Input: part model. Units: mm. Frame: model coordinates. Coordinates: 2 decimals unless noted, no trailing zeros. Order: outer loops, then holes, each group sorted by start corner. A loop starts at its lowest first (then second) coordinate and runs counter-clockwise, first axis right, second up. Notation, with made-up numbers: (-34, 54) - (15, 54) arc R8 ccw to (15, 59) - close; hole circle Ø9 at (64.25, 60.5). An arc over 180 degrees is marked (long way). One line per question, with ' | ' between items. Start each with the question number.
```python
from build123d import *

# Parameters (mm, degrees)
REVOLVE3_ANGLE      = 90
BOSS_EXTRUDE2_DEPTH = 1000
BOSS_EXTRUDE4_DEPTH = 50


with BuildPart() as part:
    # Sketch2 → Revolve3 (revolve)
    with BuildSketch(Plane.XY):
        with BuildLine():
            Line((-0.654182434, 15.02), (-10.654182434, 15.02))
            Line((-10.654182434, 15.02), (-10.654182434, 0))
            Line((-10.654182434, 0), (0, 0))
            Line((0, 0), (25.4, 0))
            Line((25.4, 0), (35.4, 0))
            Line((35.4, 0), (35.4, 4.5))
            Line((35.4, 4.5), (25.4, 4.5))
            add(Edge.make_bspline(
                [(-0.654182434, 15.02), (-0.219836229, 14.810704372), (0.610598489, 14.410982375), (2.74095302, 13.386545583), (4.34709547, 12.619135975), (6.701613478, 11.49599419), (8.606916476, 10.59589253), (10.790885987, 9.570629713), (12.810835282, 8.63757915), (14.944119423, 7.669787097), (16.950761864, 6.79193378), (18.75556814, 6.044207346), (20.238794329, 5.486207444), (21.39416777, 5.103578745), (22.215591012, 4.870934478), (22.897035956, 4.710298297), (23.464492683, 4.605633048), (23.954091395, 4.538072471), (24.354277235, 4.503624983), (24.669284768, 4.488813447), (24.918595629, 4.485402054), (25.124701431, 4.488218611), (25.279381224, 4.493757229), (25.359889237, 4.497669109), (25.4, 4.5)],
                knots=[0.083771138, 0.083771138, 0.083771138, 0.083771138, 0.083771138, 0.152014176, 0.220257214, 0.288500251, 0.356743288, 0.424986327, 0.493229366, 0.561472406, 0.629715448, 0.697958493, 0.757156968, 0.791278497, 0.81934393, 0.841893906, 0.858954658, 0.874282948, 0.887931591, 0.900718778, 0.906405686, 0.912092593, 0.917779499, 0.923466404, 0.923466404, 0.923466404, 0.923466404, 0.923466404], degree=4))
        make_face()
    revolve(axis=Axis((0, 0, 0), (1, 0, 0)), revolution_arc=REVOLVE3_ANGLE)

    # Sketch11 → Boss-Extrude2 (add)
    with BuildSketch(Plane.XY):
        with BuildLine():
            Line((25.133318649, 0), (101.333318649, 0))
            ThreePointArc((101.333318649, 0), (63.233318649, 38.1), (25.133318649, 0))
        make_face()
    extrude(amount=BOSS_EXTRUDE2_DEPTH)

    # Sketch16 → Boss-Extrude4 (add)
    with BuildSketch(Plane(origin=(0, 0, 0), x_dir=(0, 0, -1), z_dir=(1, 0, 0))):
        with BuildLine():
            Line((-967.503760297, 0), (-970.507760297, 0))
            ThreePointArc((-970.507760297, 0), (-969.005760297, 1.502), (-967.503760297, 0))
        make_face()
    extrude(amount=BOSS_EXTRUDE4_DEPTH)


solid = part.part
```
(1) Material intervals for line 1 along X through (y, z) = (3.5, 347); line 2 along Y through (x, z) = (59.5, 267.5); line 3 along Y through (x, z) = (60, 129), sorted ascending. Write a range as from..to.
(2) Section B-B (x = 51). Output: boundary loops of the cut face in (y, z), then the cut area to 3 significant figures.
(3) Section A-A (z = 776). Output: boundary loops of the cut face in (x, y), then the cut area to 3 significant figures.
(4) Section C-C (y = 29). Output: boundary loops of the cut face in (x, z).
(5) Pin query (flat end, axial travel): pin 1 (1.5 mm diameter, centred on y = 20, z = 176.5, fed in from -X); pin 2 (12 mm diameter, centred on x = 59, z = 537, fed in from +Y); pin 3 (1.2 mm diameter, centred on y = 1, z = 969, fed in from -X). Return the tip coordinate at first contact, or that it passes through.
Worked answers:
1) line 1: x = 25.29..101.17 | line 2: y = 0..37.92 | line 3: y = 0..37.96
2) outline: (0, 0) - (36.08, 0) - (36.08, 1000) - (0, 1000) - close | area: 36,100 mm²
3) outline: (25.13, 0) - (101.33, 0) arc R38.1 ccw to start | area: 2,280 mm²
4) outline: (38.52, 0) - (87.94, 0) - (87.94, 1000) - (38.52, 1000) - close
5) pin 1: stops at x = 30.35 | pin 2: stops at y = 38.1 | pin 3: stops at x = 0
